```python
from build123d import *

# Parameters (mm, degrees)
F1_DEPTH = 38.1
F3_DEPTH = 12.7
F5_ANGLE = 180
F6_DEPTH = 6.35
F8_DEPTH = 31.75


with BuildPart() as f1:
    # F0 (on Top) → F1 (new body)
    with BuildSketch(Plane.XY):
        Polygon((0, 457.2), (0, 0), (300.5368529815, 50.8), (300.5368529815, 406.4), align=None)
    extrude(amount=F1_DEPTH)

    # F2 (on face) → F3 (cut)
    with BuildSketch(Plane.XY.offset(38.1)):
        with BuildLine():
            Line((287.8368529815, 158.75), (287.8368529815, 228.6))
            Line((287.8368529815, 228.6), (287.8368529815, 298.45))
            add(Edge.make_bspline(
                [(287.8368529815, 298.45), (274.0976885543, 331.7129114168), (244.462232063, 403.4612317728), (73.3301440344, 427.7271384352), (70.74195792, 425.2940959796), (70.0230365024, 423.6438925683)],
                knots=[0, 0, 0, 0, 0.1680777292, 0.3625447701, 0.3933937659, 0.3933937659, 0.3933937659, 0.3933937659], degree=3))
            add(Edge.make_bspline(
                [(70.0230365024, 423.6438925683), (68.4355376678, 419.9999671984), (63.377452963, 404.8697109281), (68.3702936505, 402.2079819696), (73.2398539672, 399.3490471662), (77.3060373008, 399.9323880306), (160.4823825419, 386.0696943096), (229.5400089317, 324.4485337175), (224.3368529815, 260.4551017284), (224.3368529815, 228.6)],
                knots=[0.3933937659, 0.3933937659, 0.3933937659, 0.3933937659, 0.4615135128, 0.495784539, 0.5311346164, 0.5602485234, 0.6989412506, 0.848957098, 1, 1, 1, 1], degree=3))
            add(Edge.make_bspline(
                [(70.0230365024, 33.5561074317), (68.4355376678, 37.1999006103), (63.377452963, 52.3292730677), (68.3702936505, 54.9937890625), (73.2398539672, 57.8444840887), (77.3060373008, 57.3174367131), (160.4823825419, 70.0436920791), (229.5400089317, 136.9971102414), (224.3368529815, 187.5921785831), (224.3368529815, 228.6)],
                knots=[0.3933937659, 0.3933937659, 0.3933937659, 0.3933937659, 0.4615135128, 0.495784539, 0.5311346164, 0.5602485234, 0.6989412506, 0.848957098, 1, 1, 1, 1], degree=3))
            add(Edge.make_bspline(
                [(287.8368529815, 158.75), (274.0976885543, 125.4870885832), (244.462232063, 53.7388397395), (73.3301440344, 29.4726759186), (70.74195792, 31.9059638852), (70.0230365024, 33.5561074317)],
                knots=[0, 0, 0, 0, 0.1680777292, 0.3625447701, 0.3933937659, 0.3933937659, 0.3933937659, 0.3933937659], degree=3))
        make_face()
    extrude(amount=-F3_DEPTH, mode=Mode.SUBTRACT)

    # F4 (on face) → F5 (revolve, cut)
    with BuildSketch(Plane.XY.offset(38.1)):
        with BuildLine():
            ThreePointArc((268.7868529815, 228.6), (278.0862126788, 206.1493596973), (300.5368529815, 196.85))
            Line((300.5368529815, 196.85), (300.5368529815, 228.6))
            Line((300.5368529815, 228.6), (268.7868529815, 228.6))
        make_face()
    revolve(axis=Axis((284.6618529815, 228.6, 38.1), (1, 0, 0)), revolution_arc=F5_ANGLE, mode=Mode.SUBTRACT)

    # F2 (on face) → F6 (cut)
    with BuildSketch(Plane.XY.offset(38.1)):
        with BuildLine():
            add(Edge.make_bspline(
                [(70.0230365024, 33.5561074317), (59.3142063381, 30.9359426227), (37.2815163913, 25.5451316791), (12.6563049092, 26.6596121467), (0, 27.2324074148)],
                knots=[0, 0, 0, 0, 0.4860427932, 1, 1, 1, 1], degree=3))
            add(Edge.make_bspline(
                [(70.0230365024, 33.5561074317), (68.4355376678, 37.1999006103), (63.377452963, 52.3292730677), (68.3702936505, 54.9937890625), (73.2398539672, 57.8444840887), (77.3060373008, 57.3174367131), (160.4823825419, 70.0436920791), (229.5400089317, 136.9971102414), (224.3368529815, 187.5921785831), (224.3368529815, 228.6)],
                knots=[0.3933937659, 0.3933937659, 0.3933937659, 0.3933937659, 0.4615135128, 0.495784539, 0.5311346164, 0.5602485234, 0.6989412506, 0.848957098, 1, 1, 1, 1], degree=3))
            add(Edge.make_bspline(
                [(70.0230365024, 423.6438925683), (68.4355376678, 419.9999671984), (63.377452963, 404.8697109281), (68.3702936505, 402.2079819696), (73.2398539672, 399.3490471662), (77.3060373008, 399.9323880306), (160.4823825419, 386.0696943096), (229.5400089317, 324.4485337175), (224.3368529815, 260.4551017284), (224.3368529815, 228.6)],
                knots=[0.3933937659, 0.3933937659, 0.3933937659, 0.3933937659, 0.4615135128, 0.495784539, 0.5311346164, 0.5602485234, 0.6989412506, 0.848957098, 1, 1, 1, 1], degree=3))
            add(Edge.make_bspline(
                [(70.0230365024, 423.6438925683), (59.3142063381, 426.2640573773), (37.2815163913, 431.6548683209), (12.6563049092, 430.5403878533), (0, 429.9675925852)],
                knots=[0, 0, 0, 0, 0.4860427932, 1, 1, 1, 1], degree=3))
            Line((0, 429.9675925852), (0, 27.2324074148))
        make_face()
    extrude(amount=-F6_DEPTH, mode=Mode.SUBTRACT)

    # F7 (on face) → F8 (join)
    with BuildSketch(Plane.XY.offset(31.75)):
        Polygon((0, 228.6), (0, 368.3), (-254, 368.3), (-254, 88.9), (0, 88.9), align=None)
    extrude(amount=-F8_DEPTH)


solid = f1.part
```
For this review, take the finished solid that the model builds, in its own axes (mm). A direction names the side the tool comes from. Give positions to 0.01 mm unless a question says otherwise; leave off trailing zeros. Loops run counter-clockwise (first coordinate to the right, second up) from the corner with the lowest first, then second, coordinate; pieces in that order, holes last. Notation, with made-up numbers: M 25.25,53 L 39.25,53 A16 cw 39.25,74 Z; hole C 30.5,35.25 d7. An arc over 180 degrees is marked long. One line per item, written item: value. Start each with the question number.
Q1. Add section A-A (z = 17). Give the boundary of the cut face in (x, y).
Q2. For L1, parallel to X at y = 267, z = 25.5; L2, parallel to Z at x = -156, y = 307.5; L3, parallel to Z at x = 259, y = 105.5, list the stretches that pass through material, from the lowest coordinate up.
Q3. Clearance check with flat-ended pins moving along their axes: pin 1 Ø19 at (y, z) = (405, 25) entering from -X; pin 2 Ø2 at (x, z) = (-94, 24.5) entering from -Y; pin 3 Ø4 at (x, z) = (97, 12) entering from +Y. State where each tip first meets the part, or that it passes through.
Q4. Add section B-B (x = -108). Give the boundary of the cut face in (y, z), and give its area (3 significant figures).
Q5. Machinability: for faces 1 (the face through (-125, 368.3, 16)), 2 (the face through (-129, 88.9, 16)), 3 (the face through (287.837, 180, 32)), which of the approach directions +Z, -Z, +X, -X, +Y, -Y give a long, thin tool a straight path to every point of the face, cutting with its end or side? Answer none if there is none.
Reply:
1. outline: M -254,88.9 L 0,88.9 L 0,0 L 300.54,50.8 L 300.54,204.88 A23.72 cw 300.54,252.32 L 300.54,406.4 L 0,457.2 L 0,368.3 L -254,368.3 Z
2. L1: -254 to 224.57, 287.84 to 300.54
2. L2: 0 to 31.75
2. L3: 0 to 25.4
3. pin 1: x = 0
3. pin 2: y = 88.9
3. pin 3: y = 441.14
4. outline: M 88.9,0 L 368.3,0 L 368.3,31.75 L 88.9,31.75 Z
4. area: 8,870 mm²
5. face 1: +Z, -Z, -X, +Y
5. face 2: +Z, -Z, -X, -Y
5. face 3: +Z
